from build123d import *
from build123d.topology import SkipClean

# Parameters (mm, degrees)
SKETCH1_R           = 6.5
BOSS_EXTRUDE1_DEPTH = 7
SKETCH2_R           = 5
CUT_EXTRUDE1_DEPTH  = 1.5
SKETCH3_R           = 2.5
SKETCH3_W           = 3
SKETCH3_H           = 3.5
CUT_EXTRUDE2_DEPTH  = 12.554220008
BOSS_EXTRUDE2_DEPTH = 1.5


with BuildPart() as part:
    # Sketch1 → Boss-Extrude1 (new body)
    with BuildSketch(Plane(origin=(0, 0, 0), x_dir=(1, 0, 0), z_dir=(0, 1, 0))):
        with Locations(Location((0, 0, 0), (0, 0, 90))):
            Circle(SKETCH1_R)
    extrude(amount=BOSS_EXTRUDE1_DEPTH)

    # Sketch2 → Cut-Extrude1 (cut)
    with BuildSketch(Plane.XZ):
        with Locations(Location((0, 0, 0), (0, 0, 270))):
            Circle(SKETCH2_R)
    extrude(amount=-CUT_EXTRUDE1_DEPTH, mode=Mode.SUBTRACT)

    # Sketch3 → Cut-Extrude2 (cut, through all)
    with BuildSketch(Plane(origin=(0, 7, 0), x_dir=(1, 0, 0), z_dir=(0, 1, 0))):
        with Locations(Location((0, 0, 0), (0, 0, 270))):
            Circle(SKETCH3_R)
        with Locations((0, 4.95)):
            Rectangle(SKETCH3_W, SKETCH3_H)
        with Locations((0, -4.95)):
            Rectangle(SKETCH3_W, SKETCH3_H)
    extrude(amount=-CUT_EXTRUDE2_DEPTH, mode=Mode.SUBTRACT)

    # Sketch4 → Boss-Extrude2 (add)
    with SkipClean():  # the faces are left unmerged after this step: merging them gives an invalid solid
        with BuildSketch(Plane.XZ.offset(-1.5)):
            with BuildLine():
                Line((-1.5, 2), (-1.5, 3.2))
                Line((-1.5, 3.2), (1.5, 3.2))
                Line((1.5, 3.2), (1.5, 2))
                ThreePointArc((1.5, 2), (0, 2.5), (-1.5, 2))
            make_face()
            with BuildLine():
                Line((-1.5, -2), (-1.5, -3.2))
                Line((-1.5, -3.2), (1.5, -3.2))
                Line((1.5, -3.2), (1.5, -2))
                ThreePointArc((1.5, -2), (0, -2.5), (-1.5, -2))
            make_face()
        extrude(amount=BOSS_EXTRUDE2_DEPTH)
    add(part.part.scale(1), mode=Mode.REPLACE)  # the faces are merged on a copy


solid = part.part
Geometry: final body of the model. Coordinates: model frame, mm. A direction names the side the tool comes from. Give positions to 0.01 mm unless a question says otherwise; leave off trailing zeros. Write each loop counter-clockwise with the first axis right and the second up, starting at its lowest first coordinate (ties: lowest second). Pieces come first, ordered by that corner, then holes.
(1) Cut plane C-C, the plane x = 0. Return loops of the section in (y, z).
(2) Access query for faces 1 (the flat face through (1.5, 1, -3)), 2 (the flat face through (0, 7, -3)), 3 (the flat face through (-1.5, 4, -5)), 4 (the flat face through (-5.3, 0, -0.4)), 5 (the flat face through (1.5, 4, 5)). Directions: +Z, -Z, +X, -X, +Y, -Y. A direction counts if a zero-diameter tool reaches every point of the face in a straight line with its end or side. Return the directions, or none.
(3) First-contact query: P1, Ø2.5, axis at y = 3.5, z = -4.5, coming from the -X side; P2, Ø1.2, axis at x = 0.5, y = 0.5, coming from the -Z side; P3, Ø1.6, axis at y = 4, z = -5.5, coming from the +X side. Flat tips, straight axial feed; report the tip coordinate or a pass-through.
(4) Cut plane D-D, the plane y = 4.5. Return loops of the section in (x, z), then the cut area to 3 significant figures.
(5) Cut plane B-B, the plane y = 0.75. Return loops of the section in (x, z), then the cut area to 3 significant figures.
(6) Cut plane A-A, the plane z = 0. Return loops of the section in (x, y).
(7) Ray query, line 1 (X direction, y = 4, z = 0); line 2 (Z direction, x = 0, y = 5.55); line 3 (X direction, y = 3.25, z = -1.5). Return the intervals inside material, ascending.
(8) Mould query, pull axis X, two halves, no side actions, for faces 6 (the cylindrical face through (-5, 1, 0)), 7 (the flat face through (0, 0, -3)), 8 (the cylindrical face through (6.5, 3.5, 0.1)). Classes: released by +X, released by -X, zero draft, split by the parting line, or undercut.
Values follow:
1. outline: (0, -3.2) - (7, -3.2) - (7, -2.5) - (0, -2.5) - close; (0, 2.5) - (7, 2.5) - (7, 3.2) - (0, 3.2) - close
2. face 1: -Y
2. face 2: +Z, -Z, +X, -X, +Y
2. face 3: -Z, +Y, -Y
2. face 4: +Z, -Z, +X, -X, -Y
2. face 5: +Z, +Y, -Y
3. P1: stops at x = -5.63
3. P2: stops at z = -3.2
3. P3: stops at x = 4.49
4. outline: (-1.5, -6.32) - (-1.5, -3.2) - (1.5, -3.2) - (1.5, -6.32) arc R6.5 ccw to (1.5, 6.32) - (1.5, 3.2) - (-1.5, 3.2) - (-1.5, 6.32) arc R6.5 ccw to start; hole circle Ø5 at (0, 0)
4. area: 93.6 mm2
5. outline: (-1.5, -6.32) - (-1.5, -4.77) arc R5 cw to (-1.5, 4.77) - (-1.5, 6.32) arc R6.5 ccw to start; (-1.5, -3.2) - (1.5, -3.2) - (1.5, -2) arc R2.5 cw to (-1.5, -2) - close; (-1.5, 2) arc R2.5 cw to (1.5, 2) - (1.5, 3.2) - (-1.5, 3.2) - close; (1.5, -6.32) arc R6.5 ccw to (1.5, 6.32) - (1.5, 4.77) arc R5 cw to (1.5, -4.77) - close
5. area: 50.2 mm2
6. outline: (-6.5, 0) - (-5, 0) - (-5, 1.5) - (-2.5, 1.5) - (-2.5, 7) - (-6.5, 7) - close; (2.5, 1.5) - (5, 1.5) - (5, 0) - (6.5, 0) - (6.5, 7) - (2.5, 7) - close
7. line 1: x = -6.5 to -2.5, 2.5 to 6.5
7. line 2: z = -3.2 to -2.5, 2.5 to 3.2
7. line 3: x = -6.32 to -2, 2 to 6.32
8. face 6: undercut
8. face 7: zero draft
8. face 8: released by +X
